Read the model definition and answer for the solid it produces. Units are mm, in the model's axes. A direction names the side the tool comes from. Round coordinates to 2 decimals unless told otherwise and drop trailing zeros. Loops run counter-clockwise (first coordinate to the right, second up) from the corner with the lowest first, then second, coordinate; pieces in that order, holes last. Notation, with made-up numbers: (21, -37) - (54, -37) arc R26 cw to (54, -19) - close; hole circle Ø9 at (74.25, 72). An arc over 180 degrees is marked (long way). Use one line per item in the form item = value. Start each with the question number.
```python
from build123d import *

# Parameters (mm, degrees)
BOX001_W          = 1
BOX001_H          = 2
BOX001_DEPTH      = 6.4
CYLINDER003_R     = 1.6
CYLINDER003_DEPTH = 6.5
CYLINDER001_R     = 4.8
CYLINDER001_DEPTH = 6.7
CYLINDER002_R     = 3.15
CYLINDER002_DEPTH = 19
CYLINDER004_R     = 7.1
CYLINDER004_DEPTH = 3
CYLINDER_R        = 7.1
CYLINDER_DEPTH    = 3
BOX_W             = 33
BOX_H             = 94
BOX_DEPTH         = 33


with BuildPart() as slit001:
    # Box001 → Box001 (new body)
    with BuildSketch(Plane(origin=(17.5, 48, 16.8), x_dir=(1, 0, 0), z_dir=(0, 0, 1))):
        with Locations((0.5, 1)):
            Rectangle(BOX001_W, BOX001_H)
    extrude(amount=BOX001_DEPTH)


with BuildPart() as hole001:
    # Cylinder003 → Cylinder003 (new body)
    with BuildSketch(Plane(origin=(18, 55, 16.7), x_dir=(1, 0, 0), z_dir=(0, 0, 1))):
        Circle(CYLINDER003_R)
    extrude(amount=CYLINDER003_DEPTH)


with BuildPart() as shaft002:
    # Cylinder001 → Cylinder001 (new body)
    with BuildSketch(Plane(origin=(18, 73, 20), x_dir=(1, 0, 0), z_dir=(0, -1, 0))):
        Circle(CYLINDER001_R)
    extrude(amount=CYLINDER001_DEPTH)


with BuildPart() as shaft003:
    # Cylinder002 → Cylinder002 (new body)
    with BuildSketch(Plane(origin=(18, 67, 20), x_dir=(1, 0, 0), z_dir=(0, -1, 0))):
        Circle(CYLINDER002_R)
    extrude(amount=CYLINDER002_DEPTH)


with BuildPart() as shaft004:
    # Cylinder004 → Cylinder004 (new body)
    with BuildSketch(Plane(origin=(18, 69.4, 20), x_dir=(1, 0, 0), z_dir=(0, -1, 0))):
        Circle(CYLINDER004_R)
    extrude(amount=CYLINDER004_DEPTH)


with BuildPart() as obj1:
    # Cylinder → Cylinder (new body)
    with BuildSketch(Plane(origin=(18, 76, 20), x_dir=(1, 0, 0), z_dir=(0, -1, 0))):
        Circle(CYLINDER_R)
    extrude(amount=CYLINDER_DEPTH)

    # Fusion: union shaft002, shaft003, shaft004
    add(shaft002.part)
    add(shaft003.part)
    add(shaft004.part)

    # Cut: cut hole001
    add(hole001.part, mode=Mode.SUBTRACT)

    # Cut001: cut slit001
    add(slit001.part, mode=Mode.SUBTRACT)


with BuildPart() as obj1_1:
    # Cut001 placement: moved
    add(obj1.part.moved(Location((-1, 0, -3))))


with BuildPart() as cap001:
    # Box → Box (new body)
    with BuildSketch(Plane(origin=(0, 76, 0), x_dir=(1, 0, 0), z_dir=(0, 0, 1))):
        with Locations((16.5, 47)):
            Rectangle(BOX_W, BOX_H)
    extrude(amount=BOX_DEPTH)

    # Fusion001: union obj1
    add(obj1_1.part)


with BuildPart() as cap001_1:
    # Fusion001 placement: moved
    add(cap001.part.moved(Location((1, 0, 3))))


solid = cap001_1.part
```
1) Straight lines are drawn through the part: line 1 (Y direction, x = 18, z = 19.5); line 2 (Y direction, x = 9.5, z = 24.5); line 3 (X direction, y = 55, z = 21). For each, find the intervals that lie inside material, in ascending order. Write a range as from..to.
2) For faces 1 (the flat face through (17.5, 49, 20)), 2 (the flat face through (17, 170, 19)), 3 (the cylindrical face through (17.317, 57.278, 16.925)), 4 (the cylindrical face through (14.46, 71.23, 23.24)), determine the directions among +Z, -Z, +X, -X, +Y, -Y from which every point of the face is accessible in a straight line to the end or side of a thin tool.
3) Flat-ended cylindrical pins translate along their axes: pin 1 (1 mm diameter, centred on x = 6.5, z = 28.5, fed in from -Y); pin 2 (1.6 mm diameter, centred on y = 49, z = 21.5, fed in from +X); pin 3 (2 mm diameter, centred on x = 21.5, z = 26, fed in from -Y); pin 4 (10 mm diameter, centred on x = 12, z = 24.5, fed in from -Y). Find the tip coordinate at first contact, or state that the pin passes through.
4) A cutting plane is placed at D-D on y = 55. Write down the section's boundary in (x, z).
5) A cutting plane is placed at C-C on x = 9. Write down the section's boundary in (y, z), plus the area to 3 significant figures.
6) Determine the mould class of faces 5 (the flat face through (17, 124, 3)), 6 (the flat face through (34, 122, 19)), 7 (the flat face through (18.5, 49, 20)) for opening direction X: +X half, -X half, draft (parallel to the pull), parting line (faces both ways), or undercut.
7) A cutting plane is placed at B-B on z = 26. Write down the section's boundary in (x, y), plus the area to 3 significant figures.
Checks:
q1.line_1 = 50..53.4, 56.6..170
q1.line_2 = 76..170
q1.line_3 = 15.01..16.4, 19.6..20.99
q2.face_1 = +Z, -Z, -Y
q2.face_2 = +Z, -Z, +X, -X, +Y
q2.face_3 = -Y
q2.face_4 = none
q3.pin_1 = 76
q3.pin_2 = 21.07
q3.pin_3 = 66.4
q3.pin_4 = 48
q4.outline = (16.4, 17.29) - (16.4, 22.71) arc R3.15 ccw to start; (19.6, 17.29) arc R3.15 ccw to (19.6, 22.71) - close
q5.outline = (76, 3) - (170, 3) - (170, 36) - (76, 36) - close
q5.area = 3,100 mm²
q6.face_5 = draft
q6.face_6 = +X half
q6.face_7 = undercut
q7.outline = (1, 76) - (14.2, 76) - (14.2, 73) - (21.8, 73) - (21.8, 76) - (34, 76) - (34, 170) - (1, 170) - close; (14.2, 66.4) - (21.8, 66.4) - (21.8, 69.4) - (14.2, 69.4) - close
q7.area = 3,150 mm²
